Check sheet for the drawn part. Datum: minimum x, y, z corner. Units: mm. A direction names the side the tool comes from. Coordinates: 2 decimals unless noted, no trailing zeros. Write each loop counter-clockwise with the first axis right and the second up, starting at its lowest first coordinate (ties: lowest second). Pieces come first, ordered by that corner, then holes. Notation, with made-up numbers: (50, 16.5) -> (78, 16.5) arc R22 cw to (78, 23.5) -> close; hole circle Ø1 at (53.25, 67). An arc over 180 degrees is marked (long way). Write item = value, one per line. Start each with the question number.
(1) Section check B-B (x = 50). Record the cut outline in (y, z).
(2) Mould release check, pull along X, two halves, no side actions. Record for the marked faces 3 and 4: released by +X, released by -X, zero draft, split by the parting line, or undercut.
(3) Section check C-C (z = 20). Record the cut outline in (x, y).
(4) Set-up check for the marked faces 1 and 2: record each of +Z, -Z, +X, -X, +Y, -Y from which the full face is reachable in a straight line by a thin tool's end or side.
(5) Section check D-D (x = 20). Record the cut outline in (y, z), plus the area to 3 significant figures.
(6) Section check A-A (y = 3.2). Record the cut outline in (x, z), plus the area to 3 significant figures.
(7) Material ranges on probe 1 along X at (y, z) = (2.8, 20); probe 2 along X at (y, z) = (2.3, 17.5); probe 3 along Y at (x, z) = (9, 4.5), recorded low to high. Write a range as [from, to].
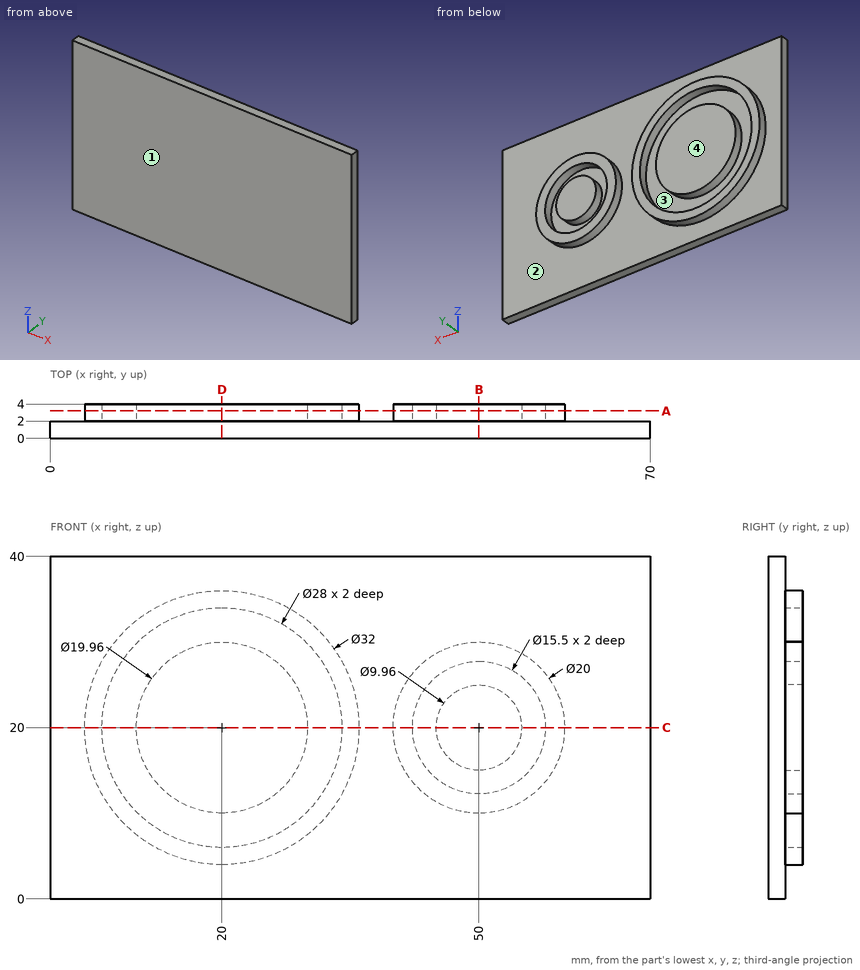
Response:
q1.outline = (0, 0) -> (2, 0) -> (2, 10) -> (4, 10) -> (4, 12.25) -> (2, 12.25) -> (2, 15.02) -> (4, 15.02) -> (4, 24.98) -> (2, 24.98) -> (2, 27.75) -> (4, 27.75) -> (4, 30) -> (2, 30) -> (2, 40) -> (0, 40) -> close
q2.face_3 = undercut
q2.face_4 = zero draft
q3.outline = (0, 0) -> (70, 0) -> (70, 2) -> (60, 2) -> (60, 4) -> (57.75, 4) -> (57.75, 2) -> (54.98, 2) -> (54.98, 4) -> (45.02, 4) -> (45.02, 2) -> (42.25, 2) -> (42.25, 4) -> (40, 4) -> (40, 2) -> (36, 2) -> (36, 4) -> (34, 4) -> (34, 2) -> (29.98, 2) -> (29.98, 4) -> (10.02, 4) -> (10.02, 2) -> (6, 2) -> (6, 4) -> (4, 4) -> (4, 2) -> (0, 2) -> close
q4.face_1 = +Z, -Z, +X, -X, -Y
q4.face_2 = +Y
q5.outline = (0, 0) -> (2, 0) -> (2, 4) -> (4, 4) -> (4, 6) -> (2, 6) -> (2, 10.02) -> (4, 10.02) -> (4, 29.98) -> (2, 29.98) -> (2, 34) -> (4, 34) -> (4, 36) -> (2, 36) -> (2, 40) -> (0, 40) -> close
q5.area = 128 mm2
q6.outline = circle Ø32 at (20, 20); circle Ø19.96 at (20, 20); circle Ø20 at (50, 20); circle Ø9.96 at (50, 20); hole circle Ø28 at (20, 20); hole circle Ø15.5 at (50, 20)
q6.area = 705 mm2
q7.probe_1 = [4, 6], [10.02, 29.98], [34, 36], [40, 42.25], [45.02, 54.98], [57.75, 60]
q7.probe_2 = [4.2, 6.23], [10.34, 29.66], [33.77, 35.8], [40.32, 42.66], [45.69, 54.31], [57.34, 59.68]
q7.probe_3 = [0, 2]
